The listing builds one solid part. Answer for the finished solid, in the listing's coordinates (mm). Coordinates: 2 decimals unless noted, no trailing zeros. Order: outer loops, then holes, each group sorted by start corner. A loop starts at its lowest first (then second) coordinate and runs counter-clockwise, first axis right, second up. Notation, with made-up numbers: (46, 29.5) - (54, 29.5) arc R24 ccw to (54, 50.5) - close; hole circle Ø3 at (17.5, -34). An arc over 180 degrees is marked (long way). Use a Markdown table: item, result. Add a question column.
Item 1: Find the intervals of material crossed by line 1 along Y through (x, z) = (20, 8.3); line 2 along X through (y, z) = (32, 0.5); line 3 along X through (y, z) = (8, 9), in increasing order.
Item 2: The part is cut by section C-C, the plane y = 20. Give the vertices of the cut face in (x, z) (3 decimals), then the cut area to 3 significant figures.
Item 3: Flat-ended cylindrical pins translate along their axes: P1, Ø2.5, axis at x = 144.5, y = 34.5, coming from the +Z side; P2, Ø2, axis at x = 146, y = 7, coming from the -Z side; P3, Ø2, axis at x = 93, y = 60, coming from the -Z side. Find the tip coordinate at first contact, or state that the pin passes through.
Item 4: The part is cut by section A-A, the plane y = 7. Give the vertices of the cut face in (x, z).
Item 5: The part is cut by section B-B, the plane x = 146. Give the vertices of the cut face in (y, z), then the cut area to 3 significant figures.
from build123d import *

# Parameters (mm, degrees)
SKETCH1_W                                        = 166
SKETCH1_H                                        = 85
BOSS_EXTRUDE3_DEPTH                              = 9.53
CBORE_FOR_M3_HEX_HEAD_MACHINE_SCREW2_D           = 3.6
CBORE_FOR_M3_HEX_HEAD_MACHINE_SCREW2_CBORE_D     = 8.4
CBORE_FOR_M3_HEX_HEAD_MACHINE_SCREW2_CBORE_DEPTH = 2.3
M4X0_7_TAPPED_HOLE1_D                            = 3.3
M4X0_7_TAPPED_HOLE1_DEPTH                        = 10.1
M4X0_7_TAPPED_HOLE1_TIP                          = 0.991420021


with BuildPart() as part:
    # Sketch1 → Boss-Extrude3 (new body)
    with BuildSketch(Plane(origin=(0, 0, 0), x_dir=(-1, 0, 0), z_dir=(0, 0, 1))):
        with Locations((-83, -42.5)):
            Rectangle(SKETCH1_W, SKETCH1_H)
    extrude(amount=BOSS_EXTRUDE3_DEPTH)

    # CBORE for M3 Hex Head Machine Screw2 (through all)
    with Locations(Plane(origin=(20, 33, 9.53), x_dir=(1, 0, 0), z_dir=(0, 0, 1))):
        with Locations((0, 0), (0, -26), (126, 0), (126, -26)):
            CounterBoreHole(CBORE_FOR_M3_HEX_HEAD_MACHINE_SCREW2_D / 2, CBORE_FOR_M3_HEX_HEAD_MACHINE_SCREW2_CBORE_D / 2, CBORE_FOR_M3_HEX_HEAD_MACHINE_SCREW2_CBORE_DEPTH)

    # M4x0.7 Tapped Hole1
    with Locations(Plane(origin=(63.065, 70, 9.53), x_dir=(1, 0, 0), z_dir=(0, 0, 1))):
        with Locations((0, 0), (0, -50), (39.87, 0), (39.87, -50)):
            Hole(M4X0_7_TAPPED_HOLE1_D / 2, depth=M4X0_7_TAPPED_HOLE1_DEPTH)
            with Locations((0, 0, -(M4X0_7_TAPPED_HOLE1_DEPTH + M4X0_7_TAPPED_HOLE1_TIP / 2))):  # 118° drill point
                Cone(0, M4X0_7_TAPPED_HOLE1_D / 2, M4X0_7_TAPPED_HOLE1_TIP, mode=Mode.SUBTRACT)


solid = part.part
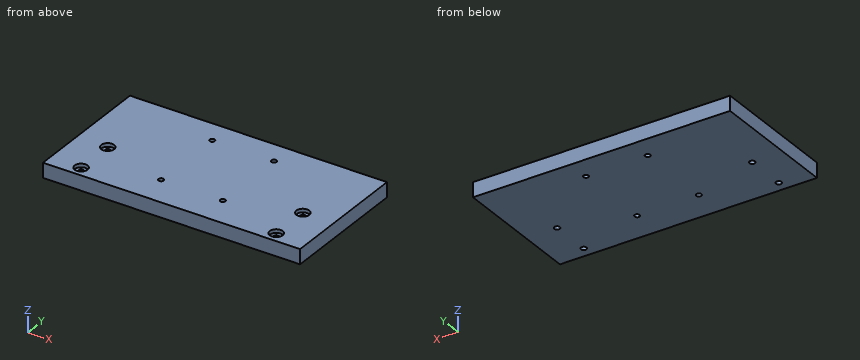
Solution:
| question | item | result |
|---|---|---|
| 1 | line 1 | y = 0 to 2.8, 11.2 to 28.8, 37.2 to 85 |
| 1 | line 2 | x = 0 to 18.5, 21.5 to 144.5, 147.5 to 166 |
| 1 | line 3 | x = 0 to 15.92, 24.08 to 141.92, 150.08 to 166 |
| 2 | outline | (0, 0) - (61.415, 0) - (61.415, 9.53) - (0, 9.53) - close; (64.715, 0) - (101.285, 0) - (101.285, 9.53) - (64.715, 9.53) - close; (104.585, 0) - (166, 0) - (166, 9.53) - (104.585, 9.53) - close |
| 2 | area | 1,520 mm2 |
| 3 | P1 | stops at z = 7.23 |
| 3 | P2 | passes through |
| 3 | P3 | stops at z = 0 |
| 4 | outline | (0, 0) - (18.2, 0) - (18.2, 7.23) - (15.8, 7.23) - (15.8, 9.53) - (0, 9.53) - close; (21.8, 0) - (144.2, 0) - (144.2, 7.23) - (141.8, 7.23) - (141.8, 9.53) - (24.2, 9.53) - (24.2, 7.23) - (21.8, 7.23) - close; (147.8, 0) - (166, 0) - (166, 9.53) - (150.2, 9.53) - (150.2, 7.23) - (147.8, 7.23) - close |
| 5 | outline | (0, 0) - (5.2, 0) - (5.2, 7.23) - (2.8, 7.23) - (2.8, 9.53) - (0, 9.53) - close; (8.8, 0) - (31.2, 0) - (31.2, 7.23) - (28.8, 7.23) - (28.8, 9.53) - (11.2, 9.53) - (11.2, 7.23) - (8.8, 7.23) - close; (34.8, 0) - (85, 0) - (85, 9.53) - (37.2, 9.53) - (37.2, 7.23) - (34.8, 7.23) - close |
| 5 | area | 719 mm2 |
